Could you check a few things on this model? Use its own coordinates, in mm. A direction names the side the tool comes from. Round coordinates to 2 decimals unless told otherwise and drop trailing zeros. Loops run counter-clockwise (first coordinate to the right, second up) from the corner with the lowest first, then second, coordinate; pieces in that order, holes last. Notation, with made-up numbers: M 5,70.25 L 46,70.25 A14 cw 46,90.25 Z; hole C 81.5,65 d7. An arc over 180 degrees is marked long. Answer in a Markdown table with one row per item.
```python
from build123d import *

# Parameters (mm, degrees)
SKETCH1_R           = 3.175
BOSS_EXTRUDE1_DEPTH = 7.62
BOSS_EXTRUDE2_DEPTH = 2.54
SKETCH6_OUTSIDE_W   = 14.587
SKETCH6_OUTSIDE_H   = 11.412
SKETCH6_OUTSIDE_R   = 2.667
CUT_EXTRUDE1_DEPTH  = 1.1938


with BuildPart() as part:
    # Sketch1 → Boss-Extrude1 (new body)
    with BuildSketch(Plane(origin=(0, 0, 0), x_dir=(1, 0, 0), z_dir=(0, 1, 0))):
        with Locations(Location((0, 0, 0), (0, 0, 90))):
            Circle(SKETCH1_R)
    extrude(amount=BOSS_EXTRUDE1_DEPTH)

    # Sketch2 → Boss-Extrude2 (add)
    with BuildSketch(Plane.XZ):
        with BuildLine():
            Line((-3.549757914, 3.175), (3.549757914, 3.175))
            ThreePointArc((3.549757914, 3.175), (4.7625, 0), (3.549757914, -3.175))
            Line((3.549757914, -3.175), (-3.549757914, -3.175))
            ThreePointArc((-3.549757914, -3.175), (-4.7625, 0), (-3.549757914, 3.175))
        make_face()
    extrude(amount=BOSS_EXTRUDE2_DEPTH)

    # Sketch6 outside → Cut-Extrude1 (cut)
    with BuildSketch(Plane(origin=(0, 5.08, 0), x_dir=(1, 0, 0), z_dir=(0, 1, 0))):
        with Locations((0.0005, 0)):
            Rectangle(SKETCH6_OUTSIDE_W, SKETCH6_OUTSIDE_H)
        with Locations(Location((0, 0, 0), (0, 0, 270))):
            Circle(SKETCH6_OUTSIDE_R, mode=Mode.SUBTRACT)
    extrude(amount=CUT_EXTRUDE1_DEPTH, mode=Mode.SUBTRACT)


solid = part.part
```
1) I want a section at C-C, the plane y = 1.5. Please give me the cut outline in (x, z) (3 decimals).
Computed:
| item | result |
|---|---|
| outline | C 0,0 d6.35 |
2) I want a section at B-B, the plane z = 0. Please give me the cut outline in (x, y) (1 decimal).
Computed:
| item | result |
|---|---|
| outline | M -4.8,-2.5 L 4.8,-2.5 L 4.8,0 L 3.2,0 L 3.2,5.1 L 2.7,5.1 L 2.7,6.3 L 3.2,6.3 L 3.2,7.6 L -3.2,7.6 L -3.2,6.3 L -2.7,6.3 L -2.7,5.1 L -3.2,5.1 L -3.2,0 L -4.8,0 Z |
3) I want a section at D-D, the plane x = -0.25. Please give me the cut outline in (y, z) (3 decimals), plus the area to 3 significant figures.
Computed:
| item | result |
|---|---|
| outline | M -2.54,-3.175 L 0,-3.175 L 0,-3.165 L 5.08,-3.165 L 5.08,-2.655 L 6.274,-2.655 L 6.274,-3.165 L 7.62,-3.165 L 7.62,3.165 L 6.274,3.165 L 6.274,2.655 L 5.08,2.655 L 5.08,3.165 L 0,3.165 L 0,3.175 L -2.54,3.175 Z |
| area | 63.1 mm² |
4) I need wall thicknesses on line 1 (Y direction, x = 2.75, z = -1.75); line 2 (X direction, y = 6, z = 0); line 3 (X direction, y = 7, z = -1). Which ranges of each line are inside material? Lowest first, please.
Computed:
| item | result |
|---|---|
| line 1 | y = -2.54 to 0 |
| line 2 | x = -2.67 to 2.67 |
| line 3 | x = -3.01 to 3.01 |
5) Will this pin go through, and if not, where does the flat tip stop? P1, Ø1, axis at y = 2, z = 2, coming from the -X side.
Computed:
| item | result |
|---|---|
| P1 | stops at x = -2.8 |
6) I want a section at A-A, the plane x = -3. Please give me the cut outline in (y, z) (3 decimals), plus the area to 3 significant figures.
Computed:
| item | result |
|---|---|
| outline | M -2.54,-3.175 L 0,-3.175 L 0,-1.04 L 5.08,-1.04 L 5.08,1.04 L 0,1.04 L 0,3.175 L -2.54,3.175 Z; M 6.274,-1.04 L 7.62,-1.04 L 7.62,1.04 L 6.274,1.04 Z |
| area | 29.5 mm² |
7) Which directions (+Z, -Z, +X, -X, +Y, -Y) give clear straight access to the entire face, cutting with the end or side of a thin tool? Please do faces 1 (the face through (-3.4, 0, 0)), 2 (the face through (-2, 5.08, -2)), 3 (the face through (3.5, 0, 0)).
Computed:
| item | result |
|---|---|
| face 1 | -X, +Y |
| face 2 | none |
| face 3 | +X, +Y |
